```python
from build123d import *

# Parameters (mm, degrees)
SKETCH1_R           = 69.85
BOSS_EXTRUDE1_DEPTH = 34.29
SKETCH5_R           = 67.30999999999999
CUT_EXTRUDE1_DEPTH  = 105.56504721942221
SKETCH6_R           = 2.539999999999996
SKETCH6_R_2         = 2.5399999999999983
SKETCH6_R_3         = 2.5400000000000005
SKETCH6_R_4         = 2.53999999999999
BOSS_EXTRUDE3_DEPTH = 36.195
SKETCH12_R          = 1.523999999999992
SKETCH12_R_2        = 1.5239999999999905
SKETCH12_R_3        = 1.523999999999989
SKETCH12_R_4        = 1.5239999999999874
CUT_EXTRUDE3_DEPTH  = 11.43
BOSS_EXTRUDE4_START = -2.54
SKETCH13_R          = 1.599999999999998
BOSS_EXTRUDE4_DEPTH = 2.54
FILLET1_R           = 2.54
CIRPATTERN2_DEPTH   = 2.54
SKETCH14_R          = 69.85
SKETCH14_R_2        = 67.30999999999997
BOSS_EXTRUDE5_DEPTH = 2.54


with BuildPart() as part:
    # Sketch1 → Boss-Extrude1 (new body)
    with BuildSketch(Plane(origin=(0, 0, 0), x_dir=(1, 0, 0), z_dir=(0, 1, 0))):
        with Locations(Location((0, 0, 0), (0, 0, 270))):
            Circle(SKETCH1_R)
    extrude(amount=BOSS_EXTRUDE1_DEPTH)

    # Sketch5 → Cut-Extrude1 (cut, through all)
    with BuildSketch(Plane(origin=(0, 34.29, 0), x_dir=(1, 0, 0), z_dir=(0, 1, 0))):
        with Locations(Location((0, 0, 0), (0, 0, 270))):
            Circle(SKETCH5_R)
    extrude(amount=-CUT_EXTRUDE1_DEPTH, mode=Mode.SUBTRACT)

    # Sketch6 → Boss-Extrude3 (add)
    with BuildSketch(Plane(origin=(0, 34.29, 0), x_dir=(1, 0, 0), z_dir=(0, 1, 0))):
        with Locations(Location((67.30999999999999, 0, 0), (0, 0, 270))):
            Circle(SKETCH6_R)
        with Locations(Location((-2.3501e-13, 67.30999999999999, 0), (0, 0, 270))):
            Circle(SKETCH6_R_2)
        with Locations(Location((-67.30999999999999, -4.7002e-13, 0), (0, 0, 270))):
            Circle(SKETCH6_R_3)
        with Locations(Location((7.0503e-13, -67.30999999999999, 0), (0, 0, 270))):
            Circle(SKETCH6_R_4)
    extrude(amount=-BOSS_EXTRUDE3_DEPTH)

    # Sketch12 → Cut-Extrude3 (cut)
    with BuildSketch(Plane(origin=(0, 34.29, 0), x_dir=(1, 0, 0), z_dir=(0, 1, 0))):
        with Locations(Location((-67.30999999999999, 0, 0), (0, 0, 270))):
            Circle(SKETCH12_R)
        with Locations(Location((2.3501e-13, 67.30999999999999, 0), (0, 0, 270))):
            Circle(SKETCH12_R_2)
        with Locations(Location((67.30999999999999, -4.7002e-13, 0), (0, 0, 270))):
            Circle(SKETCH12_R_3)
        with Locations(Location((-7.0503e-13, -67.30999999999999, 0), (0, 0, 270))):
            Circle(SKETCH12_R_4)
    extrude(amount=-CUT_EXTRUDE3_DEPTH, mode=Mode.SUBTRACT)

    # Sketch13 → Boss-Extrude4 (add)
    with BuildSketch(Plane.XZ.offset(BOSS_EXTRUDE4_START)):
        with BuildLine():
            Line((-49.35750883434136, 45.76540638591458), (-5.173661326046175, 1.5815588776185732))
            ThreePointArc((-5.173661326046175, 1.5815588776185732), (3.825447686219193, -3.825447686219249), (-1.5815588776184986, 5.173661326046197))
            Line((-1.5815588776184986, 5.173661326046197), (-45.76540638591367, 49.35750883434221))
            ThreePointArc((-45.76540638591367, 49.35750883434221), (-47.59535744166605, 47.59535744166695), (-49.35750883434136, 45.76540638591458))
        make_face()
        with Locations(Location((0, 0, 0), (0, 0, 270))):
            Circle(SKETCH13_R, mode=Mode.SUBTRACT)
    extrude(amount=BOSS_EXTRUDE4_DEPTH)

    # Fillet1
    fillet1_edges = [part.edges().sort_by_distance(p)[0] for p in [
        (-49.35750883434137, 1.27, 45.76540638591459),
        (-45.76540638591368, 1.27, 49.35750883434221),
        (-1.5815588776184981, 1.27, 5.173661326046197),
        (-5.173661326046176, 1.27, 1.5815588776185734),
    ]]
    fillet(fillet1_edges, radius=FILLET1_R)

    # CirPattern2: read off the stored shape, not the designer's step
    # CirPattern2 outline → CirPattern2 (add)
    with BuildSketch(Plane(origin=(0, 0, 0), x_dir=(1, 0, 0), z_dir=(0, 1, 0))):
        with BuildLine():
            ThreePointArc((1.581558878, 5.173661326), (3.825447686, 3.825447686), (5.173661326, 1.581558878))
            Line((5.173661326, 1.581558878), (47.454273375, 43.862170927))
            ThreePointArc((47.454273375, 43.862170927), (49.350009241, 44.604162841), (51.181709878, 43.715771456))
            ThreePointArc((51.181709878, 43.715771456), (47.595357442, 47.595357442), (43.715771456, 51.181709878))
            ThreePointArc((43.715771456, 51.181709878), (44.604162841, 49.350009241), (43.862170927, 47.454273375))
            Line((43.862170927, 47.454273375), (1.581558878, 5.173661326))
        make_face()
        with BuildLine():
            ThreePointArc((-5.173661326, 1.581558878), (-3.825447686, 3.825447686), (-1.581558878, 5.173661326))
            Line((-1.581558878, 5.173661326), (-43.862170927, 47.454273375))
            ThreePointArc((-43.862170927, 47.454273375), (-44.604162841, 49.350009241), (-43.715771456, 51.181709878))
            ThreePointArc((-43.715771456, 51.181709878), (-47.595357442, 47.595357442), (-51.181709878, 43.715771456))
            ThreePointArc((-51.181709878, 43.715771456), (-49.350009241, 44.604162841), (-47.454273375, 43.862170927))
            Line((-47.454273375, 43.862170927), (-5.173661326, 1.581558878))
        make_face()
        with BuildLine():
            Line((47.454273375, -43.862170927), (5.173661326, -1.581558878))
            ThreePointArc((5.173661326, -1.581558878), (3.825447686, -3.825447686), (1.581558878, -5.173661326))
            Line((1.581558878, -5.173661326), (43.862170927, -47.454273375))
            ThreePointArc((43.862170927, -47.454273375), (44.604162841, -49.350009241), (43.715771456, -51.181709878))
            ThreePointArc((43.715771456, -51.181709878), (47.595357442, -47.595357442), (51.181709878, -43.715771456))
            ThreePointArc((51.181709878, -43.715771456), (49.350009241, -44.604162841), (47.454273375, -43.862170927))
        make_face()
    extrude(amount=CIRPATTERN2_DEPTH)

    # Sketch14 → Boss-Extrude5 (add)
    with BuildSketch(Plane.XZ):
        with Locations(Location((0, 0, 0), (0, 0, 270))):
            Circle(SKETCH14_R)
        with Locations(Location((0, 0, 0), (0, 0, 92.162233192))):
            Circle(SKETCH14_R_2, mode=Mode.SUBTRACT)
    extrude(amount=BOSS_EXTRUDE5_DEPTH)

    # Fillet2: read off the stored shape, not the designer's step
    # Fillet2 outline → Fillet2 (revolve, cut)
    with BuildSketch(Plane.XY):
        with BuildLine():
            Line((69.85, -2.54), (69.85, -1.905))
            ThreePointArc((69.85, -1.905), (69.664012806, -2.354012806), (69.215, -2.54))
            Line((69.215, -2.54), (69.85, -2.54))
        make_face()
        with BuildLine():
            Line((67.31, -2.54), (67.945, -2.54))
            ThreePointArc((67.945, -2.54), (67.495987194, -2.354012806), (67.31, -1.905))
            Line((67.31, -1.905), (67.31, -2.54))
        make_face()
    revolve(axis=Axis((0, 0, 0), (0, 1, 0)), mode=Mode.SUBTRACT)


solid = part.part
```
Design review of the part built by this model. Coordinates are the model's own, in mm. A direction names the side the tool comes from. Coordinates: 2 decimals unless noted, no trailing zeros. Order: outer loops, then holes, each group sorted by start corner. A loop starts at its lowest first (then second) coordinate and runs counter-clockwise, first axis right, second up.
1) For faces 1 (the flat face through (-27.077, 1.288, 23.484)), 2 (the flat face through (0, 2.54, -4)), list the 3-axis set-ups (+Z, -Z, +X, -X, +Y, -Y) from which the entire face can be reached by the end or side of a thin tool; tool diameter is ignored.
2) Clearance check with flat-ended pins moving along their axes: pin 1 (3 mm diameter, centred on y = 28.5, z = 21.5, fed in from -X); pin 2 (5 mm diameter, centred on x = -21, y = 6.5, fed in from -Z); pin 3 (2.5 mm diameter, centred on x = 67.5, z = 0, fed in from +Y). State where each tip first meets the part, or that it passes through.
3) Take a section at B-B, the plane y = 29.5. Give the boundary of the cut face in (x, z), and give its area (3 significant figures).
4) Mouldability with a two-part tool opening along X and no side actions: class faces 3 (the flat face through (-22.91, 1.29, 26.5)), 4 (the flat face through (-51, -2.54, -46)) as +X half, -X half, draft (parallel to the pull), parting line (faces both ways), or undercut.
5) Take a section at A-A, the plane y = 6.5. Give the boundary of the cut face in (x, z).
6) Wall thickness on line 1 along Z through (x, y) = (-1, 29); line 2 along Z through (x, y) = (-17.5, 2); line 3 along X through (y, z) = (2, -7.5): over which ranges is each line inside the solid? List them lowest first.
7) Take a section at C-C, the plane x = 10.5. State how many separate pieces and enclosed holes the cut face has, and give its area (3 significant figures).
Returned:
1. face 1: +Y, -Y
1. face 2: +Y
2. pin 1: stops at x = -66.93
2. pin 2: stops at z = -67.36
2. pin 3: stops at y = 22.86
3. outline: circle Ø139.7 at (0, 0); hole circle Ø3.05 at (-67.31, 0); hole (-67.26, -2.54) arc R67.31 ccw to (-2.54, -67.26) arc R2.54 cw to (2.54, -67.26) arc R67.31 ccw to (67.26, -2.54) arc R2.54 cw to (67.26, 2.54) arc R67.31 ccw to (2.54, 67.26) arc R2.54 cw to (-2.54, 67.26) arc R67.31 ccw to (-67.26, 2.54) arc R2.54 cw to start; hole circle Ø3.05 at (0, -67.31); hole circle Ø3.05 at (0, 67.31); hole circle Ø3.05 at (67.31, 0)
3. area: 1,110 mm2
4. face 3: undercut
4. face 4: draft
5. outline: circle Ø139.7 at (0, 0); hole (-67.26, -2.54) arc R67.31 ccw to (-2.54, -67.26) arc R2.54 cw to (2.54, -67.26) arc R67.31 ccw to (67.26, -2.54) arc R2.54 cw to (67.26, 2.54) arc R67.31 ccw to (2.54, 67.26) arc R2.54 cw to (-2.54, 67.26) arc R67.31 ccw to (-67.26, 2.54) arc R2.54 cw to start
6. line 1: z = -69.84 to -68.46, -66.16 to -64.98, 64.98 to 66.16, 68.46 to 69.84
6. line 2: z = -67.62 to -65, -21.09 to -13.91, 13.91 to 21.09, 65 to 67.62
6. line 3: x = -69.45 to -66.89, -11.09 to -3.91, 3.91 to 11.09, 66.89 to 69.45
7. separate pieces: 4
7. enclosed holes: 0
7. area: 225 mm2
